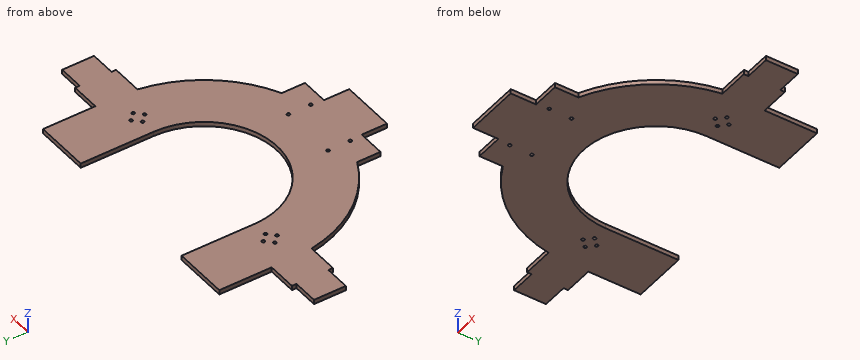
from build123d import *

# Parameters (mm, degrees)
BOSS_EXTRUDE1_DEPTH     = 3.175
SKETCH3_R               = 2.152500013
CUT_EXTRUDE2_DEPTH      = 343.063448214
CUT_EXTRUDE3_DEPTH      = 343.019240291
CUT_EXTRUDE3_DEPTH_BACK = 343.019240291
SKETCH4_R               = 2.159


with BuildPart() as part:
    # Sketch1 → Boss-Extrude1 (new, symmetric)
    with BuildSketch(Plane.XY):
        with BuildLine():
            Line((-101.800000108, 0), (-101.800000108, 101.6))
            Line((-101.800000108, 101.6), (-178.000000108, 101.6))
            Line((-178.000000108, 101.6), (-178.000000108, 28.575))
            Line((-178.000000108, 28.575), (-218.874999892, 28.575))
            Line((-218.874999892, 28.575), (-218.874999892, 22.225))
            Line((-218.874999892, 22.225), (-254.200000108, 22.225))
            Line((-254.200000108, 22.225), (-254.200000108, -22.225))
            Line((-254.200000108, -22.225), (-218.874999892, -22.225))
            Line((-218.874999892, -22.225), (-218.874999892, -28.575))
            Line((-218.874999892, -28.575), (-175.691403926, -28.575))
            ThreePointArc((-175.691403926, -28.575), (-142.258508697, -106.98839536), (-76.2, -160.865036719))
            Line((-76.2, -160.865036719), (-76.2, -193.474999892))
            Line((-76.2, -193.474999892), (-38.1, -193.474999892))
            Line((-38.1, -193.474999892), (-38.1, -228.800000108))
            Line((-38.1, -228.800000108), (38.1, -228.800000108))
            Line((38.1, -228.800000108), (38.1, -193.474999892))
            Line((38.1, -193.474999892), (76.2, -193.474999892))
            Line((76.2, -193.474999892), (76.2, -160.865036719))
            ThreePointArc((76.2, -160.865036719), (142.258508697, -106.98839536), (175.691403926, -28.575))
            Line((175.691403926, -28.575), (218.874999892, -28.575))
            Line((218.874999892, -28.575), (218.874999892, -22.225))
            Line((218.874999892, -22.225), (254.200000108, -22.225))
            Line((254.200000108, -22.225), (254.200000108, 22.225))
            Line((254.200000108, 22.225), (218.874999892, 22.225))
            Line((218.874999892, 22.225), (218.874999892, 28.575))
            Line((218.874999892, 28.575), (178.000000108, 28.575))
            Line((178.000000108, 28.575), (178.000000108, 101.6))
            Line((178.000000108, 101.6), (101.800000108, 101.6))
            Line((101.800000108, 101.6), (101.800000108, 0))
            ThreePointArc((101.800000108, 0), (0, -101.800000108), (-101.800000108, 0))
        make_face()
    extrude(amount=BOSS_EXTRUDE1_DEPTH, both=True)

    # Sketch3 → Cut-Extrude2 (cut, through all)
    with BuildSketch(Plane.XY.offset(3.175)):
        with Locations((-133.6, 9.5)):
            Circle(SKETCH3_R)
        with Locations((-124.1, 0)):
            Circle(SKETCH3_R)
        with Locations((-143.1, 0)):
            Circle(SKETCH3_R)
        with Locations((-133.6, -9.5)):
            Circle(SKETCH3_R)
        with Locations(Location((133.6, -9.5, 0), (0, 0, 180))):
            Circle(SKETCH3_R)
        with Locations(Location((143.1, 0, 0), (0, 0, 180))):
            Circle(SKETCH3_R)
        with Locations(Location((124.1, 0, 0), (0, 0, 180))):
            Circle(SKETCH3_R)
        with Locations(Location((133.6, 9.5, 0), (0, 0, 180))):
            Circle(SKETCH3_R)
    extrude(amount=-CUT_EXTRUDE2_DEPTH, mode=Mode.SUBTRACT)

    # Sketch4 → Cut-Extrude3 (cut, two sides: drawn at the far end of the back side and taken through both)
    with BuildSketch(Plane.XY.offset(-CUT_EXTRUDE3_DEPTH_BACK)):
        with Locations((40, -145.365036719)):
            Circle(SKETCH4_R)
        with Locations((-40, -145.365036719)):
            Circle(SKETCH4_R)
        with Locations((-40, -176.365036719)):
            Circle(SKETCH4_R)
        with Locations((40, -176.365036719)):
            Circle(SKETCH4_R)
    extrude(amount=CUT_EXTRUDE3_DEPTH + CUT_EXTRUDE3_DEPTH_BACK, mode=Mode.SUBTRACT)


solid = part.part
Here's how the part is built. I have some questions about the finished solid (model axes, mm). Coordinates: 2 decimals unless noted, no trailing zeros. Write each loop counter-clockwise with the first axis right and the second up, starting at its lowest first coordinate (ties: lowest second). Pieces come first, ordered by that corner, then holes.
Item 1: Will these pins go through, and if not, where does the flat tip stop? pin 1 (1.5 mm diameter, centred on y = -48.5, z = 0, fed in from +X); pin 2 (5.5 mm diameter, centred on x = 133.6, y = -9.5, fed in from +Z) (3 decimals); pin 3 (1.9 mm diameter, centred on y = -183, z = 0, fed in from +X); pin 4 (1.9 mm diameter, centred on y = 58, z = -1, fed in from -X).
Item 2: I want a section at C-C on x = 86. Write out the boundary of the cut face in (y, z) (3 decimals), and give its area (3 significant figures).
Item 3: I want a section at D-D on z = -1. Count the separate pieces of the cut face and the enclosed holes in it, and give its area (3 significant figures).
Item 4: If I drill on line 1 (X direction, y = 76, z = 3); line 2 (Y direction, x = 133.6, z = 0.5); line 3 (X direction, y = -94.5, z = -0.5), over which ranges is the centre line in solid material (lowest first)?
Item 5: I want a section at B-B on y = -90. Write out the boundary of the cut face in (x, z) (3 decimals), and give its area (3 significant figures).
Item 6: I want a section at A-A on y = 37. Write out the boundary of the cut face in (x, z) (3 decimals), and give its area (3 significant figures).
Findings below:
1. pin 1: stops at x = 171.48
1. pin 2: stops at z = 3.175
1. pin 3: stops at x = 76.2
1. pin 4: stops at x = -178
2. outline: (-155.846, -3.175) - (-54.472, -3.175) - (-54.472, 3.175) - (-155.846, 3.175) - close
2. area: 644 mm2
3. separate pieces: 1
3. enclosed holes: 12
3. area: 62,600 mm2
4. line 1: x = -178 to -101.8, 101.8 to 178
4. line 2: y = -117.62 to -11.65, -7.35 to 7.35, 11.65 to 101.6
4. line 3: x = -150.84 to -37.85, 37.85 to 150.84
5. outline: (-153.571, -3.175) - (-47.574, -3.175) - (-47.574, 3.175) - (-153.571, 3.175) - close; (47.574, -3.175) - (153.571, -3.175) - (153.571, 3.175) - (47.574, 3.175) - close
5. area: 1,350 mm2
6. outline: (-178, -3.175) - (-101.8, -3.175) - (-101.8, 3.175) - (-178, 3.175) - close; (101.8, -3.175) - (178, -3.175) - (178, 3.175) - (101.8, 3.175) - close
6. area: 968 mm2
